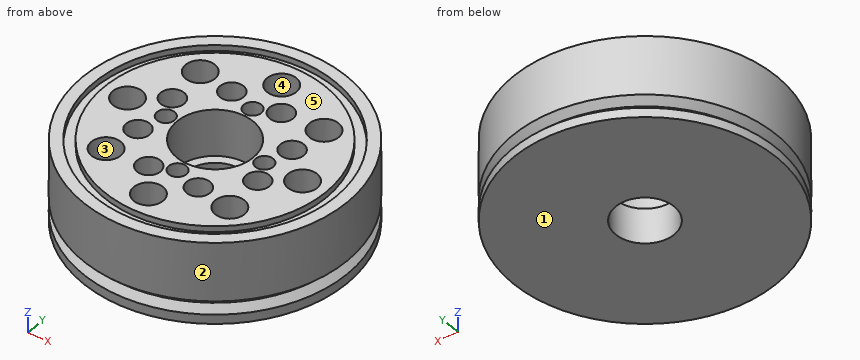
from build123d import *

# Parameters (mm, degrees)
SKETCH_1_R               = 22.5
EXTRUDE_1_DEPTH          = 14
SKETCH_4_R               = 20.533551365
SKETCH_4_R_2             = 18.873819988
CUT_EXTRUDE_2_DEPTH      = 1
SKETCH_5_R               = 6.5
CUT_EXTRUDE_3_DEPTH      = 8
SKETCH_6_R               = 5
CUT_EXTRUDE_4_DEPTH      = 8
SKETCH_7_R               = 1.5
CUT_EXTRUDE_5_DEPTH      = 5
PATTERN_CIRCULAR_1_COUNT = 4
SKETCH_8_R               = 2.5
CUT_EXTRUDE_6_DEPTH      = 5
PATTERN_CIRCULAR_2_COUNT = 8
SKETCH_9_R               = 2
CUT_EXTRUDE_10_DEPTH     = 5
PATTERN_CIRCULAR_3_COUNT = 8
SCALE_1_SCALE            = 1.2444444


with BuildPart() as part:
    # 草图1 → 凸台-拉伸1 (new body)
    with BuildSketch(Plane.XY):
        Circle(SKETCH_1_R)
    extrude(amount=EXTRUDE_1_DEPTH)

    # 草图4 → 切除-拉伸2 (cut)
    with BuildSketch(Plane.XY.offset(14)):
        Circle(SKETCH_4_R)
        Circle(SKETCH_4_R_2, mode=Mode.SUBTRACT)
    extrude(amount=-CUT_EXTRUDE_2_DEPTH, mode=Mode.SUBTRACT)

    # 草图5 → 切除-拉伸3 (cut)
    with BuildSketch(Plane.XY.offset(14)):
        Circle(SKETCH_5_R)
    extrude(amount=-CUT_EXTRUDE_3_DEPTH, mode=Mode.SUBTRACT)

    # 草图6 → 切除-拉伸4 (cut)
    with BuildSketch(Plane.XY.offset(6)):
        Circle(SKETCH_6_R)
    extrude(amount=-CUT_EXTRUDE_4_DEPTH, mode=Mode.SUBTRACT)

    # 草图7 → 切除-拉伸5 (cut)
    with BuildSketch(Plane.XY.offset(14)):
        with Locations((0, 8.372803667)):
            Circle(SKETCH_7_R)
    cut_extrude_5 = extrude(amount=-CUT_EXTRUDE_5_DEPTH, mode=Mode.SUBTRACT)

    # 阵列(圆周)1: 切除-拉伸5 ×4 about axis
    pattern_circular_1_axis = Axis((0, 0, 0), (0, 0, 1))
    for i in range(1, PATTERN_CIRCULAR_1_COUNT):
        add(cut_extrude_5.rotate(pattern_circular_1_axis, i * 360 / PATTERN_CIRCULAR_1_COUNT), mode=Mode.SUBTRACT)

    # 草图8 → 切除-拉伸6 (cut)
    with BuildSketch(Plane.XY.offset(14)):
        with Locations((0, 14.876496216)):
            Circle(SKETCH_8_R)
    cut_extrude_6 = extrude(amount=-CUT_EXTRUDE_6_DEPTH, mode=Mode.SUBTRACT)

    # 阵列(圆周)2: 切除-拉伸6 ×8 about axis
    pattern_circular_2_axis = Axis((0, 0, 0), (0, 0, 1))
    for i in range(1, PATTERN_CIRCULAR_2_COUNT):
        add(cut_extrude_6.rotate(pattern_circular_2_axis, i * 360 / PATTERN_CIRCULAR_2_COUNT), mode=Mode.SUBTRACT)

    # 草图9 → 切除-拉伸10 (cut)
    with BuildSketch(Plane.XY.offset(14)):
        with Locations((-4.513696744, 9.661753254)):
            Circle(SKETCH_9_R)
    cut_extrude_10 = extrude(amount=-CUT_EXTRUDE_10_DEPTH, mode=Mode.SUBTRACT)

    # 阵列(圆周)3: 切除-拉伸10 ×8 about axis
    pattern_circular_3_axis = Axis((0, 0, 0), (0, 0, 1))
    for i in range(1, PATTERN_CIRCULAR_3_COUNT):
        add(cut_extrude_10.rotate(pattern_circular_3_axis, i * 360 / PATTERN_CIRCULAR_3_COUNT), mode=Mode.SUBTRACT)


with BuildPart() as part_1:
    # 缩放比例1: scaled about (0, 0, 6.525153491)
    add(part.part.scale(SCALE_1_SCALE).moved(Location((0, 0, -1.59503723))))

    # 草图10 → 切除-旋转1 (revolve, cut)
    with BuildSketch(Plane(origin=(0, 0, 0), x_dir=(0, 0, -1), z_dir=(1, 0, 0))):
        Polygon((-0.40004552, 28.00491625), (-1.828401218, 26.576560552), (-3.256756916, 28.00491625), align=None)
    revolve(axis=Axis((0, 0, 0), (0, 0, 1)), mode=Mode.SUBTRACT)


solid = part_1.part
Build history of the part. All positions in model axes, mm. Face numbers are marked on the shaded views. A direction names the side the tool comes from. Round coordinates to 2 decimals unless told otherwise and drop trailing zeros. Write each loop counter-clockwise with the first axis right and the second up, starting at its lowest first coordinate (ties: lowest second). Pieces come first, ordered by that corner, then holes. Notation, with made-up numbers: (73.25, -36) - (121.25, -36) arc R9 cw to (121.25, -20) - close; hole circle Ø10 at (63.5, 70). An arc over 180 degrees is marked (long way). Use CSV: the item, a comma, the result in double quotes.
(1) Pin check, flat tips, straight feed: P1, Ø1.5, axis at y = -6.5, z = 12, coming from the -X side; P2, Ø6, axis at x = -8, z = 13, coming from the -Y side; P3, Ø3, axis at x = -12.47, y = 4.53, coming from the +Z side; P4, Ø6.5, axis at x = 4.53, y = 12.47, coming from the +Z side. Stop position of each tip, or through.
Response:
P1,"x = -27.4"
P2,"y = -27.55"
P3,"z = 9.6"
P4,"z = 15.83"
(2) Wall check: line 1 (Y direction, x = -9.5, z = 15); line 2 (X direction, y = -11.5, z = 12); line 3 (Y direction, x = 17.5, z = 15). Give the ranges that are in metal, low to high.
Response:
line 1,"-26.34 to -23.72, -21.48 to -1.62, 1.62 to 21.48, 23.72 to 26.34"
line 2,"-25.53 to -15.76, -10.42 to -6.82, -2.24 to -1.52, 1.52 to 3.18, 8.05 to 10.42, 15.76 to 25.53"
line 3,"-21.86 to -18.62, -15.67 to -2.94, 2.94 to 15.67, 18.62 to 21.86"
(3) Mould opens along Y. For the marked faces 1, 2 and 3 say: pulls with the +Y half, pulls with the -Y half, needs draft (parallel to the pull), parting line crosses it, or undercut.
Response:
face 1,"needs draft"
face 2,"parting line crosses it"
face 3,"undercut"
(4) Band-saw the part on A-A (z = 7.5). Write the cut outline in (x, y).
Response:
outline,"circle Ø56 at (0, 0); hole circle Ø16.18 at (0, 0)"
(5) 3-axis set-ups, long thin cutter, end or side, ignore diameter. For the marked faces 4 and 5: which of +Z, -Z, +X, -X, +Y, -Y reach the whole face in a straight line?
Response:
face 4,"+Z"
face 5,"+Z, +X, -X, +Y, -Y"
